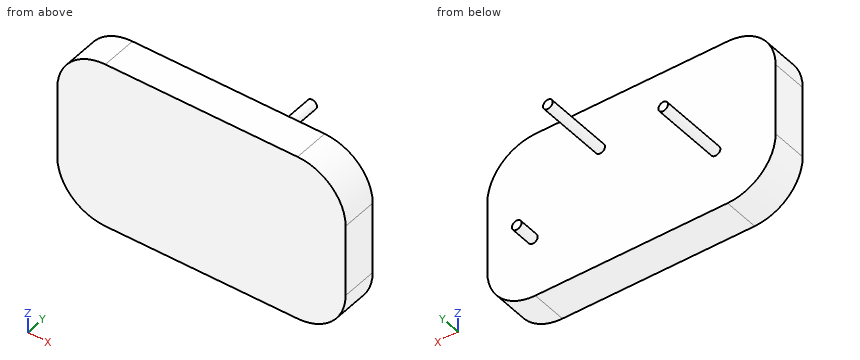
from build123d import *

# Parameters (mm, degrees)
SKETCH1_W           = 120
SKETCH1_H           = 70
BOSS_EXTRUDE1_DEPTH = 15
FILLET1_R           = 20
SKETCH2_R           = 2
BOSS_EXTRUDE3_DEPTH = 9
SKETCH6_R           = 2
BOSS_EXTRUDE4_DEPTH = 20


with BuildPart() as part:
    # Sketch1 → Boss-Extrude1 (new body)
    with BuildSketch(Plane(origin=(0, 0, 0), x_dir=(1, 0, 0), z_dir=(0, 1, 0))):
        with Locations((60, 35)):
            Rectangle(SKETCH1_W, SKETCH1_H)
    extrude(amount=BOSS_EXTRUDE1_DEPTH)

    # Fillet1
    fillet1_edges = [part.edges().sort_by_distance(p)[0] for p in [
        (0, 7.5, -70),
        (120, 7.5, -70),
        (120, 7.5, 0),
        (0, 7.5, 0),
    ]]
    fillet(fillet1_edges, radius=FILLET1_R)

    # Sketch2 → Boss-Extrude3 (add)
    with BuildSketch(Plane(origin=(0, 15, 0), x_dir=(1, 0, 0), z_dir=(0, 1, 0))):
        with Locations(Location((25, 45, 0), (0, 0, 90))):
            Circle(SKETCH2_R)
        with Locations(Location((73, 20, 0), (0, 0, 90))):
            Circle(SKETCH2_R)
        with Locations(Location((101, 45, 0), (0, 0, 90))):
            Circle(SKETCH2_R)
    extrude(amount=BOSS_EXTRUDE3_DEPTH)

    # Sketch6 → Boss-Extrude4 (add)
    with BuildSketch(Plane(origin=(0, 24, 0), x_dir=(1, 0, 0), z_dir=(0, 1, 0))):
        with Locations(Location((25, 45, 0), (0, 0, 90))):
            Circle(SKETCH6_R)
        with Locations(Location((73, 20, 0), (0, 0, 90))):
            Circle(SKETCH6_R)
    extrude(amount=BOSS_EXTRUDE4_DEPTH)


solid = part.part
Read the model definition and answer for the solid it produces. Units are mm, in the model's axes. Give positions to 0.01 mm unless a question says otherwise; leave off trailing zeros. Write each loop counter-clockwise with the first axis right and the second up, starting at its lowest first coordinate (ties: lowest second). Pieces come first, ordered by that corner, then holes. Notation, with made-up numbers: (43.25, 20) - (82.25, 20) arc R4 ccw to (82.25, 27) - close; hole circle Ø11 at (-24.5, -39.75). An arc over 180 degrees is marked (long way). Use CSV: the item, a comma, the result in double quotes. Start each with the question number.
(1) Find section B-B (x = 25). Give the vertices of the cut face in (y, z).
(2) Find section D-D (z = -62). Give the vertices of the cut face in (x, y).
(3) Find section C-C (z = -45). Give the vertices of the cut face in (x, y), plus the area to 3 significant figures.
(4) Given P1, Ø4, axis at x = 99.5, z = -45, coming from the +Y side; P2, Ø2, axis at y = 17, z = -52.5, coming from the +X side; P3, Ø21, axis at x = 70, z = -29, coming from the +Y side, each flat-ended and moving along its own axis, determine where each tip first touches the part or whether it passes through.
(5) Find section A-A (y = 5). Give the vertices of the cut face in (x, z), plus the area to 3 significant figures.
(6) Consider line 1 along Y through (x, z) = (69.5, -66); line 2 along Z through (x, y) = (74, 20); line 3 along Z through (x, y) = (17, 3). Determine where each line is inside the solid, lowest interval first.
Findings below:
1,outline,"(0, -70) - (15, -70) - (15, -47) - (44, -47) - (44, -43) - (15, -43) - (15, 0) - (0, 0) - close"
2,outline,"(4, 0) - (116, 0) - (116, 15) - (4, 15) - close"
3,outline,"(0, 0) - (120, 0) - (120, 15) - (103, 15) - (103, 24) - (99, 24) - (99, 15) - (27, 15) - (27, 44) - (23, 44) - (23, 15) - (0, 15) - close"
3,area,"1,950 mm2"
4,P1,"y = 24"
4,P2,"through"
4,P3,"y = 44"
5,outline,"(0, -50) arc R20 ccw to (20, -70) - (100, -70) arc R20 ccw to (120, -50) - (120, -20) arc R20 ccw to (100, 0) - (20, 0) arc R20 ccw to (0, -20) - close"
5,area,"8,060 mm2"
6,line 1,"0 to 15"
6,line 2,"-21.73 to -18.27"
6,line 3,"-69.77 to -0.23"
